Read the model definition and answer for the solid it produces. Units are mm, in the model's axes. Face numbers are marked on the shaded views. A direction names the side the tool comes from. Coordinates: 2 decimals unless noted, no trailing zeros. Order: outer loops, then holes, each group sorted by start corner. A loop starts at its lowest first (then second) coordinate and runs counter-clockwise, first axis right, second up. Notation, with made-up numbers: (8, -2) -> (55, -2) arc R15 ccw to (55, 20) -> close; hole circle Ø2 at (-10.5, 47.25). An arc over 180 degrees is marked (long way). Use CSV: the item, a comma, the result in double quotes.
Autodesk Inventor part; units mm, degrees
ref_plane "Start plane" through (0, 0, 0) normal (0, 0, 1) x (1, 0, 0)
ref_plane "End plane" through (0, 0, 1000) normal (0, 0, 1) x (1, 0, 0)
ref_plane "YZ Plane" through (0, 0, 0) normal (1, 0, 0) x (0, 1, 0)
ref_plane "Start plane" through (0, 0, 0) normal (0, 0, 1) x (1, 0, 0)
ref_plane "End plane" through (0, 0, 1000) normal (0, 0, 1) x (1, 0, 0)
sketch "Sketch" plane through (0, 0, 0) normal (0, 0, 1) x (1, 0, 0)
  line L0 (-40, -34) -> (-40, 34)
  line L1 (-34, 40) -> (34, 40)
  line L2 (40, 34) -> (40, -34)
  line L3 (34, -40) -> (-34, -40)
  arc A0 (-40, -34) -> (-34, -40) centre (-34, -34) ccw
  arc A1 (40, 34) -> (34, 40) centre (34, 34) ccw
  arc A2 (-34, 40) -> (-40, 34) centre (-34, 34) ccw
  arc A3 (34, -40) -> (40, -34) centre (34, -34) ccw
  arc A4 (-34, 37) -> (-37, 34) centre (-34, 34) ccw
  line L4 (-34, 37) -> (34, 37)
  arc A5 (37, 34) -> (34, 37) centre (34, 34) ccw
  line L5 (37, 34) -> (37, -34)
  arc A6 (34, -37) -> (37, -34) centre (34, -34) ccw
  line L6 (34, -37) -> (-34, -37)
  arc A7 (-37, -34) -> (-34, -37) centre (-34, -34) ccw
  line L7 (-37, -34) -> (-37, 34)
  line L8 (0, 44.3196) -> (0, -44.3196) construction
  line L9 (-1340.2663, 0) -> (380.2663, 0) construction
  dimension "d7" = 6
  dimension "d9" = 80
  dimension "d11" = 80
  dimension "d12" = 3
  dimension "d15" = 40
  dimension "d16" = 40
extrude "Body" add sketch "Sketch" along normal up to surface (1000 mm away) from surface at 0
sketch "Sketch3" plane through (0, 0, 0) normal (0, 0, 1) x (1, 0, 0)
  line L0 (0, 0) -> (10, 0)
ref_plane "Work Plane3" through (0, 0, 0) normal (0, -1, 0) x (1, 0, 0)
sketch "Sketch5" plane through (0, 0, 0) normal (0, 1, 0) x (-1, 0, 0)
  line L0 (-40, 0) -> (-40, 1000)
  line L1 (40, 0) -> (40, 1000)
  line L2 (40, 0) -> (40, 1000)
  line L3 (40, 397.5702) -> (490, 397.5702) construction
  line L4 (-47.0166, 436.8676) -> (1027.0166, 436.8676) construction
  arc A0 (-47.0166, 436.8676) -> (490, 310) centre (490, 1510) ccw construction
  line L5 (-110, 538.8152) -> (1090, 538.8152) construction
  arc A1 (-110, 538.8152) -> (-47.0166, 436.8676) centre (4, 538.8152) ccw construction
  arc A2 (1027.0166, 436.8676) -> (1090, 538.8152) centre (976, 538.8152) ccw
  line L6 (-110, 538.8152) -> (-110, 578.8152)
  line L7 (1090, 538.8152) -> (1090, 578.8152)
  line L8 (-110, 578.8152) -> (490, 578.8152) construction
  line L9 (490, 578.8152) -> (490, 0)
  arc A3 (490, 310) -> (1027.0166, 436.8676) centre (490, 1510) ccw
  line L10 (490, 578.8152) -> (1090, 578.8152)
  point P0 (0, 0)
  dimension "d22" = 450
  dimension "d24" = 1200
  dimension "d25" = 114
  dimension "d26" = 40
  dimension "d27" = 1200
  dimension "d28" = 310
  dimension "d30" = 397.5702
sketch "Sketch6" plane through (0, 0, 0) normal (0, 1, 0) x (-1, 0, 0)
  line L0 (40, 0) -> (40, 1000)
  line L1 (40, 0) -> (40, 1000)
  line L2 (-40, 0) -> (-40, 1000)
  line L3 (-40, 0) -> (-40, 1000)
  line L4 (34, 1000) -> (40, 1000)
  line L5 (40, 1000) -> (-40, 1000)
  line L6 (-40, 433.3849) -> (40, 397.5702)
  arc A0 (-47.0166, 436.8676) -> (490, 310) centre (490, 1510) ccw construction
  line L7 (40, 386.6139) -> (-40, 422.4286)
  point P0 (0, 0)
  point P1 (40, 386.6139)
  dimension "d33" = 10
extrude "Extrusion2" cut sketch "Sketch6" along normal through all both and the other way through all
sketch "Sketch4" plane through (0, 0, 0) normal (0, -1, 0) x (1, 0, 0)
  line L0 (-1340.2663, 0) -> (380.2663, 0)
  line L1 (-1340.2663, 1000) -> (380.2663, 1000)
  dimension "d18" = 1000
equation "\"d7\" = G_IR"
equation "\"d9\" = G_W"
equation "\"d11\" = G_H"
equation "\"d12\" = G_T"
equation "\"d15\" = 0.5 * d9"
equation "\"d16\" = 0.5 * d11"
equation "\"d3\" = G_L"
equation "\"d24\" = d27"
equation "\"d25\" = 0.095 * d27"
equation "\"G_W\" = 80"
equation "\"G_H\" = 80"
equation "\"G_T\" = 3"
equation "\"G_IR\" = 6"
equation "\"G_L\" = d18"
equation "\"G_OFFSET_START\" = 0"
equation "\"G_OFFSET_END\" = 0"
properties part number "ANP 1781 Leg tube" material "Steel, Mild"
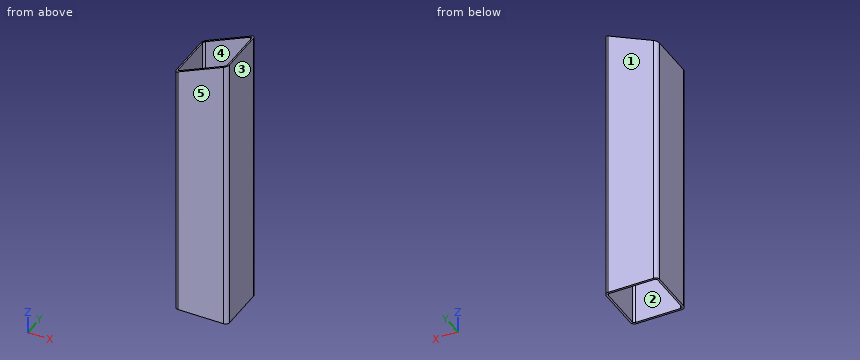
Item 1: Find section B-B, the plane z = 305. Give the vertices of the cut face in (x, y), then the cut area to 3 significant figures.
Return value:
outline,"(-40, -34) arc R6 ccw to (-34, -40) -> (34, -40) arc R6 ccw to (40, -34) -> (40, 34) arc R6 ccw to (34, 40) -> (-34, 40) arc R6 ccw to (-40, 34) -> close; hole (-37, -34) arc R3 ccw to (-34, -37) -> (34, -37) arc R3 ccw to (37, -34) -> (37, 34) arc R3 ccw to (34, 37) -> (-34, 37) arc R3 ccw to (-37, 34) -> close"
area,"901 mm^2"
Item 2: A tool of negligible diameter and unlimited length cuts with its end or side. For the marked faces 4 and 5, from which of +Z, -Z, +X, -X, +Y, -Y can it reach the whole face along a straight path? Write none if from no direction.
Return value:
face 4,"+Z, -Z"
face 5,"+Z, -Z, +X, -X, -Y"
Item 3: Find section A-A, the plane x = -26. Give the vertices of the cut face in (y, z), then the cut area to 3 significant figures.
Return value:
outline,"(-40, 0) -> (-37, 0) -> (-37, 392.88) -> (-40, 392.88) -> close; (37, 0) -> (40, 0) -> (40, 392.88) -> (37, 392.88) -> close"
area,"2,360 mm^2"
Item 4: Find section C-C, the plane y = -13. Give the vertices of the cut face in (x, z), then the cut area to 3 significant figures.
Return value:
outline,"(-40, 0) -> (-37, 0) -> (-37, 387.96) -> (-40, 386.61) -> close; (37, 0) -> (40, 0) -> (40, 422.43) -> (37, 421.09) -> close"
area,"2,430 mm^2"
Item 5: Straight lines are drawn through the part: line 1 along Y through (x, z) = (3.5, 214.5); line 2 along Y through (x, z) = (-35, 52.5). For each, find the intervals that lie inside material, in ascending order.
Return value:
line 1,"y = -40 to -37, 37 to 40"
line 2,"y = -39.92 to -36.83, 36.83 to 39.92"
Item 6: The mould has two halves that part along Y. Classify the marked faces 1, 2 and 3: +Y half, -Y half, draft (parallel to the pull), parting line (faces both ways), or undercut.
Return value:
face 1,"+Y half"
face 2,"undercut"
face 3,"draft"
